For this review, take the finished solid that the model builds, in its own axes (mm). Coordinates: 2 decimals unless noted, no trailing zeros. Loops run counter-clockwise (first coordinate to the right, second up) from the corner with the lowest first, then second, coordinate; pieces in that order, holes last. Notation, with made-up numbers: (29.25, 2.5) - (70.25, 2.5) arc R34 cw to (70.25, 35.5) - close; hole circle Ø4 at (51, 4). An arc over 180 degrees is marked (long way). One line per item, written item: value. Start each with the question number.
1. Take a section at B-B, the plane x = -1. Count the separate pieces of the cut face and the enclosed holes in it, and give its area (3 significant figures).
2. To check wall thickness, follow line 1 (X direction, y = 6.5, z = 3.5); line 2 (X direction, y = 67, z = 3); line 3 (Y direction, x = 4.5, z = 3.25). State the ranges of each line that lie inside material, in increasing order. Write a range as from..to.
3. The part is to be moulded in two halves that separate along Y. For faces 1 (the face through (-0.54, 12.56, 4.93)), 2 (the face through (-5, -1, 5)), 3 (the face through (-0.33, -2.52, 4.93)), 4 (the face through (0, -100, 5)), say which applies: released by +Y, released by -Y, zero draft, split by the parting line, or undercut.
4. Take a section at A-A, the plane y = 45. State the section outline as (x, z) points, and give its area (3 significant figures).
5. Insertion check: pin 1 (4.5 mm diameter, centred on x = 0, y = 25, fed in from +Z); pin 2 (6 mm diameter, centred on x = -2, y = -68.5, fed in from -Z). Each pin has a flat end and moves straight along its axis. Give the tip position at first contact, or say it passes through.
```python
from build123d import *

# Parameters (mm, degrees)
ESQUISSE1_W             = 10
ESQUISSE1_H             = 200
ESQUISSE1_R             = 2.5
BASE_DEPTH              = 10
ESQUISSE4_R             = 2.5
ENL_V_MAT_EXTRU_2_DEPTH = 101.995049384


with BuildPart() as part:
    # Esquisse1 → BASE (new body)
    with BuildSketch(Plane.XY):
        Rectangle(ESQUISSE1_W, ESQUISSE1_H)
        with Locations((0, 95)):
            Circle(ESQUISSE1_R, mode=Mode.SUBTRACT)
        with Locations((0, 85)):
            Circle(ESQUISSE1_R, mode=Mode.SUBTRACT)
        with Locations((0, 75)):
            Circle(ESQUISSE1_R, mode=Mode.SUBTRACT)
        with Locations((0, 65)):
            Circle(ESQUISSE1_R, mode=Mode.SUBTRACT)
        with Locations((0, 55)):
            Circle(ESQUISSE1_R, mode=Mode.SUBTRACT)
        with Locations((0, 45)):
            Circle(ESQUISSE1_R, mode=Mode.SUBTRACT)
        with Locations((0, 35)):
            Circle(ESQUISSE1_R, mode=Mode.SUBTRACT)
        with Locations((0, 25)):
            Circle(ESQUISSE1_R, mode=Mode.SUBTRACT)
        with Locations((0, 15)):
            Circle(ESQUISSE1_R, mode=Mode.SUBTRACT)
        with Locations((0, 5)):
            Circle(ESQUISSE1_R, mode=Mode.SUBTRACT)
        with Locations((0, -5)):
            Circle(ESQUISSE1_R, mode=Mode.SUBTRACT)
        with Locations((0, -15)):
            Circle(ESQUISSE1_R, mode=Mode.SUBTRACT)
        with Locations((0, -25)):
            Circle(ESQUISSE1_R, mode=Mode.SUBTRACT)
        with Locations((0, -35)):
            Circle(ESQUISSE1_R, mode=Mode.SUBTRACT)
        with Locations((0, -45)):
            Circle(ESQUISSE1_R, mode=Mode.SUBTRACT)
        with Locations((0, -55)):
            Circle(ESQUISSE1_R, mode=Mode.SUBTRACT)
        with Locations((0, -65)):
            Circle(ESQUISSE1_R, mode=Mode.SUBTRACT)
    extrude(amount=BASE_DEPTH)

    # Esquisse4 → Enlèv. mat.-Extru.2 (cut, through all)
    with BuildSketch(Plane.ZY.offset(5)):
        with Locations(Location((5, -95, 0), (0, 0, 270))):
            Circle(ESQUISSE4_R)
        with Locations(Location((5, -85, 0), (0, 0, 270))):
            Circle(ESQUISSE4_R)
        with Locations(Location((5, -75, 0), (0, 0, 270))):
            Circle(ESQUISSE4_R)
    extrude(amount=-ENL_V_MAT_EXTRU_2_DEPTH, mode=Mode.SUBTRACT)


solid = part.part
```
Solutions:
1. separate pieces: 18
1. enclosed holes: 3
1. area: 1,160 mm2
2. line 1: -5..-2, 2..5
2. line 2: -5..-1.5, 1.5..5
2. line 3: -100..-96.79, -93.21..-86.79, -83.21..-76.79, -73.21..100
3. face 1: undercut
3. face 2: zero draft
3. face 3: undercut
3. face 4: released by -Y
4. outline: (-5, 0) - (-2.5, 0) - (-2.5, 10) - (-5, 10) - close; (2.5, 0) - (5, 0) - (5, 10) - (2.5, 10) - close
4. area: 50.0 mm2
5. pin 1: through
5. pin 2: z = 0
